```python
from build123d import *

# Parameters (mm, degrees)
BOSS_EXTRUDE1_DEPTH = 15.875
SKETCH2_R           = 9.525
CUT_EXTRUDE1_DEPTH  = 218.612378382
SKETCH3_W           = 76.2
SKETCH3_H           = 6.35
SKETCH3_W_2         = 12.7
SKETCH3_H_2         = 25.4
BOSS_EXTRUDE2_DEPTH = 15.875
SKETCH9_R           = 22.225
CUT_EXTRUDE4_DEPTH  = 218.612378382
CUT_EXTRUDE6_DEPTH  = 218.612378382
BOSS_EXTRUDE3_DEPTH = 15.875
SKETCH15_R          = 1.27
CUT_EXTRUDE8_DEPTH  = 218.612378382
SKETCH13_R          = 3.126994
CUT_EXTRUDE9_DEPTH  = 218.612378382
CUT_EXTRUDE10_DEPTH = 218.612378382


with BuildPart() as part:
    # Sketch1 → Boss-Extrude1 (new body)
    with BuildSketch(Plane(origin=(0, 0, 0), x_dir=(0, 0, -1), z_dir=(1, 0, 0))):
        with BuildLine():
            ThreePointArc((57.15, 81.28), (21.180615335, 49.546911859), (-25.4, 38.1))
            Line((-25.4, 38.1), (-76.2, 38.1))
            Line((-76.2, 38.1), (-76.2, 44.45))
            Line((-76.2, 44.45), (-127, 44.45))
            Line((-127, 44.45), (-127, 38.1))
            Line((-127, 38.1), (-165.1, 38.1))
            Line((-165.1, 38.1), (-165.1, -38.1))
            Line((-165.1, -38.1), (177.8, -38.1))
            Line((177.8, -38.1), (139.7, 38.1))
            Line((139.7, 38.1), (139.7, 124.46))
            ThreePointArc((139.7, 124.46), (93.119384665, 113.013088141), (57.15, 81.28))
        make_face()
    extrude(amount=BOSS_EXTRUDE1_DEPTH)

    # Sketch2 → Cut-Extrude1 (cut, through all)
    with BuildSketch(Plane(origin=(15.875, 0, 0), x_dir=(0, 0, -1), z_dir=(1, 0, 0))):
        with Locations((111.125, 82.55)):
            Circle(SKETCH2_R)
    extrude(amount=-CUT_EXTRUDE1_DEPTH, mode=Mode.SUBTRACT)

    # Sketch3 → Boss-Extrude2 (add)
    with BuildSketch(Plane(origin=(15.875, 0, 0), x_dir=(0, 0, -1), z_dir=(1, 0, 0))):
        with Locations((114.3, -41.275)):
            Rectangle(SKETCH3_W, SKETCH3_H)
        with Locations((-63.5, -41.275)):
            Rectangle(SKETCH3_W, SKETCH3_H)
        with Locations((-171.45, 0)):
            Rectangle(SKETCH3_W_2, SKETCH3_H_2)
    extrude(amount=-BOSS_EXTRUDE2_DEPTH)

    # Sketch9 → Cut-Extrude4 (cut, through all)
    with BuildSketch(Plane(origin=(15.875, 0, 0), x_dir=(0, 0, -1), z_dir=(1, 0, 0))):
        with Locations((-19.05, 0)):
            Circle(SKETCH9_R)
    extrude(amount=-CUT_EXTRUDE4_DEPTH, mode=Mode.SUBTRACT)

    # Sketch12 → Cut-Extrude6 (cut, through all)
    with BuildSketch(Plane(origin=(15.875, 0, 0), x_dir=(0, 0, -1), z_dir=(1, 0, 0))):
        Polygon((139.7, 9.701936686), (139.7, -25.4), (157.250968343, -25.4), align=None)
        Polygon((109.05604179, 15.875), (127, -13.283932092), (127, 45.033932092), align=None)
        Polygon((119.54395821, -25.4), (101.6, 3.758932092), (83.65604179, -25.4), align=None)
        Polygon((76.2, -13.283932092), (94.14395821, 15.875), (76.2, 45.033932092), align=None)
        Polygon((83.65604179, 57.15), (101.6, 27.991067908), (119.54395821, 57.15), align=None)
        Polygon((-57.15, -18.203333333), (-57.15, 18.203333333), (-91.28125, 0), align=None)
        Polygon((-70.64375, -25.4), (-104.775, -7.196666667), (-138.90625, -25.4), align=None)
        Polygon((-152.4, -18.203333333), (-118.26875, 0), (-152.4, 18.203333333), align=None)
        Polygon((-104.775, 7.196666667), (-70.64375, 25.4), (-138.90625, 25.4), align=None)
    extrude(amount=-CUT_EXTRUDE6_DEPTH, mode=Mode.SUBTRACT)

    # Sketch14 → Boss-Extrude3 (add)
    with BuildSketch(Plane(origin=(15.875, 0, 0), x_dir=(0, 0, -1), z_dir=(1, 0, 0))):
        Polygon((147.390774674, 22.718450651), (170.109225326, -22.718450651), (175.788837989, -19.87864432), (153.070387337, 25.558256983), align=None)
    extrude(amount=-BOSS_EXTRUDE3_DEPTH)

    # Sketch15 → Cut-Extrude8 (cut, through all)
    with BuildSketch(Plane(origin=(15.875, 0, 0), x_dir=(0, 0, -1), z_dir=(1, 0, 0))):
        with Locations((-166.14759319, -13.417947427)):
            Circle(SKETCH15_R)
        with Locations((-127.867535363, 39.027514093)):
            Circle(SKETCH15_R)
        with Locations((-102.468735692, -39.026389927)):
            Circle(SKETCH15_R)
        with Locations((75.20280066, -38.886443562)):
            Circle(SKETCH15_R)
        with Locations((153.276127819, -39.019402004)):
            Circle(SKETCH15_R)
        with Locations((-24.501616142, -38.997667224)):
            Circle(SKETCH15_R)
        with Locations((-166.09635678, 13.487510741)):
            Circle(SKETCH15_R)
        with Locations((-75.205348286, 38.8896632)):
            Circle(SKETCH15_R)
        with Locations((171.314053114, -23.120059914)):
            Circle(SKETCH15_R)
        with Locations((147.792383937, 23.92327844)):
            Circle(SKETCH15_R)
    extrude(amount=-CUT_EXTRUDE8_DEPTH, mode=Mode.SUBTRACT)

    # Sketch13 → Cut-Extrude9 (cut, through all)
    with BuildSketch(Plane(origin=(15.875, 0, 0), x_dir=(0, 0, -1), z_dir=(1, 0, 0))):
        with Locations((31.75, -25.4)):
            Circle(SKETCH13_R)
        with Locations((19.05, -25.4)):
            Circle(SKETCH13_R)
        with Locations((44.45, -25.4)):
            Circle(SKETCH13_R)
        with Locations((57.15, -25.4)):
            Circle(SKETCH13_R)
        with Locations((19.05, -12.7)):
            Circle(SKETCH13_R)
        with Locations((31.75, -12.7)):
            Circle(SKETCH13_R)
        with Locations((44.45, -12.7)):
            Circle(SKETCH13_R)
        with Locations((57.15, -12.7)):
            Circle(SKETCH13_R)
        with Locations((19.05, 0)):
            Circle(SKETCH13_R)
        with Locations((31.75, 0)):
            Circle(SKETCH13_R)
        with Locations((44.45, 0)):
            Circle(SKETCH13_R)
        with Locations((57.15, 0)):
            Circle(SKETCH13_R)
        with Locations((19.05, 12.7)):
            Circle(SKETCH13_R)
        with Locations((31.75, 12.7)):
            Circle(SKETCH13_R)
        with Locations((44.45, 12.7)):
            Circle(SKETCH13_R)
        with Locations((57.15, 12.7)):
            Circle(SKETCH13_R)
        with Locations((19.05, 25.4)):
            Circle(SKETCH13_R)
        with Locations((31.75, 25.4)):
            Circle(SKETCH13_R)
        with Locations((44.45, 25.4)):
            Circle(SKETCH13_R)
        with Locations((57.15, 25.4)):
            Circle(SKETCH13_R)
        with Locations((31.75, 38.1)):
            Circle(SKETCH13_R)
        with Locations((44.45, 38.1)):
            Circle(SKETCH13_R)
        with Locations((57.15, 38.1)):
            Circle(SKETCH13_R)
        with Locations((57.15, 50.8)):
            Circle(SKETCH13_R)
    extrude(amount=-CUT_EXTRUDE9_DEPTH, mode=Mode.SUBTRACT)

    # Sketch17 → Cut-Extrude10 (cut, through all)
    with BuildSketch(Plane(origin=(15.875, 0, 0), x_dir=(0, 0, -1), z_dir=(1, 0, 0))):
        Polygon((60.325, 69.85), (85.725, 69.85), (85.725, 95.25), align=None)
    extrude(amount=-CUT_EXTRUDE10_DEPTH, mode=Mode.SUBTRACT)


solid = part.part
```
CAD build for the part. Positions are in the model's coordinates, mm. A direction names the side the tool comes from. Coordinates: 2 decimals unless noted, no trailing zeros. Order: outer loops, then holes, each group sorted by start corner. A loop starts at its lowest first (then second) coordinate and runs counter-clockwise, first axis right, second up. Notation, with made-up numbers: (7.25, -23.75) -> (32.25, -23.75) arc R36 cw to (32.25, 15.25) -> close; hole circle Ø2 at (42, 25.5). An arc over 180 degrees is marked (long way). Use one line per item in the form item = value. Start each with the question number.
1) Drop flat-ended pins along their axis: pin 1 (8 mm diameter, centred on x = 9.5, z = 134.5, fed in from -Y); pin 2 (5 mm diameter, centred on x = 7.5, y = 41.5, fed in from +Z); pin 3 (8 mm diameter, centred on x = 8.5, y = 80, fed in from +Z). Give the stop position or say it passes through.
2) Drill centre lines: L1, parallel to Z at x = 3.5, y = 20; L2, parallel to Y at x = 5.5, z = -19.05; L3, parallel to Y at x = 2.5, z = -114.5. Where is each one in solid material? Low to high. Write a range as [from, to].
3) Band-saw the part on B-B on x = 10.75. State how many separate pieces and enclosed holes the cut face has, then the cut area to 3 significant figures.
4) Tool access for faces 1 (the flat face through (8, 16, -76.2)), 2 (the flat face through (8, -38.1, 135)): list every direction of +Z, -Z, +X, -X, +Y, -Y with a clear straight run to the whole face (end or side of a thin tool).
5) Band-saw the part on C-C on z = 123. Give the cut face in (x, y) (3 decimals).
6) Pull direction Z, two halves, no side cores. Call faces 3 (the flat face through (8, -26, 165.1)), 4 (the cylindrical face through (8.049, 25.537, -41.326)), 5 (the flat face through (8, 2.5, -164.6)): +Z half, -Z half, draft (parallel to the pull), parting line (faces both ways), or undercut.
7) Band-saw the part on A-A on z = 33. Give the cut face in (x, y) (3 decimals), then the cut area to 3 significant figures.
8) Band-saw the part on D-D on z = -67.5. Give the cut face in (x, y) (3 decimals), then the cut area to 3 significant figures.
Entries:
q1.pin_1 = -38.1
q1.pin_2 = 127
q1.pin_3 = -53.22
q2.L1 = [-155.85, -127], [-111.59, -91.61], [-76.2, 9.36], [28.74, 80.77], [128.78, 165.1]
q2.L2 = [-38.1, -28.53], [-22.27, -15.83], [-9.57, -3.13], [3.13, 9.57], [15.83, 22.27], [28.53, 48.46]
q2.L3 = [-44.45, -25.4], [-17.2, 7.03], [24.72, 48.95], [57.15, 73.64], [91.46, 121.25]
q3.separate_pieces = 1
q3.enclosed_holes = 36
q3.area = 25,900 mm2
q4.face_1 = +X, -X
q4.face_2 = +Z, +X, -X, -Y
q5.outline = (0, -38.1) -> (15.875, -38.1) -> (15.875, -25.4) -> (0, -25.4) -> close; (0, -16.917) -> (15.875, -16.917) -> (15.875, -2.523) -> (0, -2.523) -> close; (0, 2.523) -> (15.875, 2.523) -> (15.875, 16.917) -> (0, 16.917) -> close; (0, 25.4) -> (15.875, 25.4) -> (15.875, 44.45) -> (0, 44.45) -> close
q6.face_3 = +Z half
q6.face_4 = undercut
q6.face_5 = -Z half
q7.outline = (0, -44.45) -> (15.875, -44.45) -> (15.875, -17.302) -> (0, -17.302) -> close; (0, 17.302) -> (15.875, 17.302) -> (15.875, 38.1) -> (0, 38.1) -> close
q7.area = 761 mm2
q8.outline = (0, -38.1) -> (15.875, -38.1) -> (15.875, 69.85) -> (0, 69.85) -> close; (0, 77.025) -> (15.875, 77.025) -> (15.875, 93.869) -> (0, 93.869) -> close
q8.area = 1,980 mm2
